```python
from build123d import *

# Parameters (mm, degrees)
SKETCH1_W                                     = 15.4
SKETCH1_H                                     = 6
BOSS_EXTRUDE1_DEPTH                           = 28
TAP_DRILL_FOR_M4X0_7_TAP1_D                   = 3.3
TAP_DRILL_FOR_M4X0_7_TAP1_DEPTH               = 13.4
TAP_DRILL_FOR_M4X0_7_TAP1_TIP                 = 0.991420021
CUT_EXTRUDE_PRESS_FIT_HOLE_FOR_SOLENOID_REACH = 31.653
SKETCH4_R                                     = 5.2
TAP_DRILL_FOR_M4X0_7_TAP2_D                   = 3.3
TAP_DRILL_FOR_M4X0_7_TAP2_DEPTH               = 3
TAP_DRILL_FOR_M4X0_7_TAP2_TIP                 = 0.991420021


with BuildPart() as part:
    # Sketch1 → Boss-Extrude1 (new body)
    with BuildSketch(Plane(origin=(0, 0, 0), x_dir=(1, 0, 0), z_dir=(0, 1, 0))):
        Rectangle(SKETCH1_W, SKETCH1_H)
    extrude(amount=BOSS_EXTRUDE1_DEPTH)

    # Tap Drill for M4x0.7 Tap1
    with Locations(Plane(origin=(-4.7, 28, 0), x_dir=(0, 0, 1), z_dir=(0, 1, 0))):
        with Locations((0, 0), (0, 9.4)):
            Hole(TAP_DRILL_FOR_M4X0_7_TAP1_D / 2, depth=TAP_DRILL_FOR_M4X0_7_TAP1_DEPTH)
            with Locations((0, 0, -(TAP_DRILL_FOR_M4X0_7_TAP1_DEPTH + TAP_DRILL_FOR_M4X0_7_TAP1_TIP / 2))):  # 118° drill point
                Cone(0, TAP_DRILL_FOR_M4X0_7_TAP1_D / 2, TAP_DRILL_FOR_M4X0_7_TAP1_TIP, mode=Mode.SUBTRACT)

    # Sketch4 → Cut-Extrude Press Fit hole for solenoid tube (cut, up to next)
    with BuildSketch(Plane.XY.offset(3), mode=Mode.PRIVATE) as cut_extrude_press_fit_hole_for_solenoid_sk1:
        with Locations((0, 8)):
            Circle(SKETCH4_R)
    cut_extrude_press_fit_hole_for_solenoid_tool1 = extrude(cut_extrude_press_fit_hole_for_solenoid_sk1.sketch, amount=-CUT_EXTRUDE_PRESS_FIT_HOLE_FOR_SOLENOID_REACH, mode=Mode.PRIVATE) & part.part
    add(cut_extrude_press_fit_hole_for_solenoid_tool1.solids().sort_by_distance((0, 8, 3))[0], mode=Mode.SUBTRACT)

    # Tap Drill for M4x0.7 Tap2
    with Locations(Plane(origin=(0, 0, 0), x_dir=(-1, 0, 0), z_dir=(0, -1, 0))):
        with Locations((-4.7, 0), (4.7, 0)):
            Hole(TAP_DRILL_FOR_M4X0_7_TAP2_D / 2, depth=TAP_DRILL_FOR_M4X0_7_TAP2_DEPTH)
            with Locations((0, 0, -(TAP_DRILL_FOR_M4X0_7_TAP2_DEPTH + TAP_DRILL_FOR_M4X0_7_TAP2_TIP / 2))):  # 118° drill point
                Cone(0, TAP_DRILL_FOR_M4X0_7_TAP2_D / 2, TAP_DRILL_FOR_M4X0_7_TAP2_TIP, mode=Mode.SUBTRACT)


solid = part.part
```
Check sheet for the modelled part. Datum: model origin and axes. Units: mm. A direction names the side the tool comes from. Coordinates: 2 decimals unless noted, no trailing zeros. Loops run counter-clockwise (first coordinate to the right, second up) from the corner with the lowest first, then second, coordinate; pieces in that order, holes last.
1) Sectioned sample at B-B (x = -0.75). Record the boundary of the cut face in (y, z), and give its area (3 significant figures).
2) Access from +Z, -Z, +X, -X, +Y, -Y to the whole of each face (thin tool, end or side, straight path). Record for faces 1 (the face through (-6.3, 21.2, 0.4)), 2 (the face through (0, 0, 0)), 3 (the face through (-3.126, 1.521, -0.496)).
3) Release check for a two-part mould opening along Z. For faces 4 (the face through (4.4, 3.8, -0.1)), 5 (the face through (0, 28, 0)), 6 (the face through (0, 14, 3)), 7 (the face through (6.336, 21.206, 0.215)) record: released by +Z, released by -Z, zero draft, split by the parting line, or undercut.
4) Material ranges on probe 1 along Z at (x, y) = (-4.7, 23.75); probe 2 along Y at (x, z) = (0, -2.45); probe 3 along X at (y, z) = (3.5, -0.45), recorded low to high.
5) Sectioned sample at A-A (y = 17.75). Record the boundary of the cut face in (x, z).
6) Gauge pin test, flat ends, axial feed: pin 1 (2 mm diameter, centred on x = -4.7, z = 0, fed in from -Y); pin 2 (6 mm diameter, centred on x = 0, y = 8, fed in from +Z); pin 3 (2 mm diameter, centred on x = 4.7, z = 0, fed in from +Y). Record the tip position at first contact, or that the pin passes through.
7) Sectioned sample at C-C (y = 7). Record the boundary of the cut face in (x, z), and give its area (3 significant figures).
Check sheet entries:
1. outline: (0, -3) - (2.85, -3) - (2.85, 3) - (0, 3) - close; (13.15, -3) - (28, -3) - (28, 3) - (13.15, 3) - close
1. area: 106 mm2
2. face 1: +Y
2. face 2: +Z, -Z, +X, -X, -Y
2. face 3: -Y
3. face 4: undercut
3. face 5: zero draft
3. face 6: released by +Z
3. face 7: undercut
4. probe 1: z = -3 to -1.65, 1.65 to 3
4. probe 2: y = 0 to 2.8, 13.2 to 28
4. probe 3: x = -7.7 to -5.38, -4.02 to -2.61, 2.61 to 4.02, 5.38 to 7.7
5. outline: (-7.7, -3) - (7.7, -3) - (7.7, 3) - (-7.7, 3) - close; hole circle Ø3.3 at (-4.7, 0); hole circle Ø3.3 at (4.7, 0)
6. pin 1: stops at y = 3.39
6. pin 2: passes through
6. pin 3: stops at y = 14.21
7. outline: (-7.7, -3) - (-5.1, -3) - (-5.1, 3) - (-7.7, 3) - close; (5.1, -3) - (7.7, -3) - (7.7, 3) - (5.1, 3) - close
7. area: 31.2 mm2
